The listing builds one solid part. Answer for the finished solid, in the listing's coordinates (mm). Face numbers are marked on the shaded views. A direction names the side the tool comes from. Give positions to 0.01 mm unless a question says otherwise; leave off trailing zeros. Loops run counter-clockwise (first coordinate to the right, second up) from the corner with the lowest first, then second, coordinate; pieces in that order, holes last. Notation, with made-up numbers: (43.25, -24) - (56.25, -24) arc R25 ccw to (56.25, 2) - close; hole circle Ø1 at (16, 72). An arc over 180 degrees is marked (long way). Write each question's results on one line, items separated by ' | '.
from build123d import *

# Parameters (mm, degrees)
F0_W     = 70
F0_H     = 22
F1_DEPTH = 78.994
F2_T     = -2
F3_W     = 13
F3_H     = 10
F3_W_2   = 8
F4_DEPTH = 25.4
F5_W     = 47
F5_H     = 4
F6_DEPTH = 25.4
F8_D     = 3


with BuildPart() as f1:
    # F0 (on Front) → F1 (new body)
    with BuildSketch(Plane.XZ):
        Rectangle(F0_W, F0_H)
    extrude(amount=F1_DEPTH)

    # F2
    f2_openings = [f1.faces().sort_by_distance(p)[0] for p in [
        (0, -39.497, 11),
    ]]
    offset(amount=F2_T, openings=f2_openings)

    # F3 (on face) → F4 (cut)
    with BuildSketch(Plane.XZ.offset(78.994)):
        with Locations((-11.289247, -0.486001)):
            Rectangle(F3_W, F3_H)
        with Locations((18.5, -0.492737)):
            Rectangle(F3_W_2, F3_H)
    extrude(amount=-F4_DEPTH, mode=Mode.SUBTRACT)

    # F5 (on face) → F6 (cut)
    with BuildSketch(Plane(origin=(-35, 0, 0), x_dir=(0, -1, 0), z_dir=(-1, 0, 0))):
        with Locations((26.5, 3.065218)):
            Rectangle(F5_W, F5_H)
    extrude(amount=-F6_DEPTH, mode=Mode.SUBTRACT)

    # F8 (through all)
    with Locations(Plane(origin=(0, 0, -11), x_dir=(1, 0, 0), z_dir=(0, 0, -1))):
        with Locations((-7.398465, 4.346834), (20.601535, 4.346834), (24.640625, 56.574557), (-22.482722, 56.045765)):
            Hole(F8_D / 2)


solid = f1.part
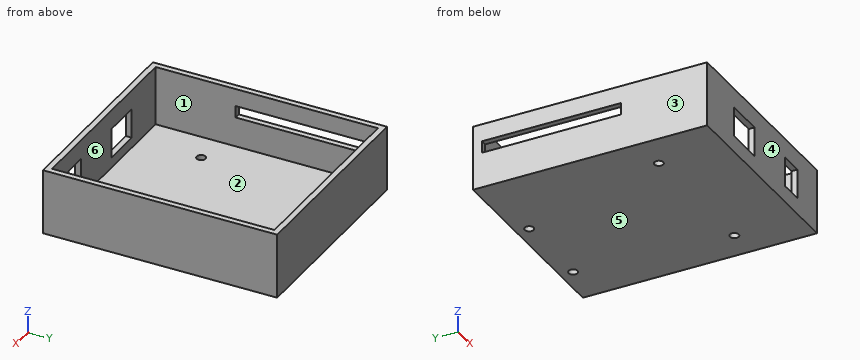
Item 1: A cutting plane is placed at A-A, the plane z = -2.5. Determine the outline of the cut face in (x, y), plus the area to 3 significant figures.
Values found:
outline: (-35, -78.99) - (-17.79, -78.99) - (-17.79, -76.99) - (-33, -76.99) - (-33, -2) - (33, -2) - (33, -76.99) - (22.5, -76.99) - (22.5, -78.99) - (35, -78.99) - (35, 0) - (-35, 0) - close; (-4.79, -78.99) - (14.5, -78.99) - (14.5, -76.99) - (-4.79, -76.99) - close | area: 538 mm²
Item 2: For the marked faces 5 and 6, determine the directions among +Z, -Z, +X, -X, +Y, -Y from which every point of the face is accessible in a straight line to the end or side of a thin tool.
Values found:
face 5: -Z, +X, -X, +Y, -Y | face 6: +Z
Item 3: A cutting plane is placed at D-D, the plane z = 2. Determine the outline of the cut face in (x, y).
Values found:
outline: (-35, -78.99) - (-17.79, -78.99) - (-17.79, -76.99) - (-33, -76.99) - (-33, -50) - (-35, -50) - close; (-35, -3) - (-33, -3) - (-33, -2) - (33, -2) - (33, -76.99) - (22.5, -76.99) - (22.5, -78.99) - (35, -78.99) - (35, 0) - (-35, 0) - close; (-4.79, -78.99) - (14.5, -78.99) - (14.5, -76.99) - (-4.79, -76.99) - close
Item 4: Find the intervals of material crossed by line 1 along X through (y, z) = (-21, 1); line 2 along Y through (x, z) = (22.5, 9.25); line 3 along Z through (x, y) = (11, -37.5), in increasing order. Write a range as [from, to].
Values found:
line 1: x = [-35, -33], [33, 35] | line 2: y = [-78.99, -76.99], [-2, 0] | line 3: z = [-11, -9]
Item 5: A cutting plane is placed at B-B, the plane x = 17. Determine the outline of the cut face in (y, z).
Values found:
outline: (-78.99, -11) - (0, -11) - (0, 11) - (-2, 11) - (-2, -9) - (-76.99, -9) - (-76.99, -5.49) - (-78.99, -5.49) - close; (-78.99, 4.51) - (-76.99, 4.51) - (-76.99, 11) - (-78.99, 11) - close
Item 6: For a pull along X with two mould halves and no side action, classify the marked faces 1, 2, 3 and 4 as released by +X, released by -X, zero draft, split by the parting line, or undercut.
Values found:
face 1: undercut | face 2: undercut | face 3: released by -X | face 4: zero draft
Item 7: A cutting plane is placed at C-C, the plane y = -47. Determine the outline of the cut face in (x, z).
Values found:
outline: (-35, -11) - (35, -11) - (35, 11) - (33, 11) - (33, -9) - (-33, -9) - (-33, 1.07) - (-35, 1.07) - close; (-35, 5.07) - (-33, 5.07) - (-33, 11) - (-35, 11) - close
